Drawing for the job (mm, zero at the part's lowest x, y, z). A direction names the side the tool comes from. Give positions to 0.01 mm unless a question says otherwise; leave off trailing zeros. Loops run counter-clockwise (first coordinate to the right, second up) from the corner with the lowest first, then second, coordinate; pieces in that order, holes last. Notation, with made-up numbers: (67.25, 5.25) -> (71.25, 5.25) arc R22 ccw to (71.25, 18.25) -> close; hole circle Ø7 at (-2.75, 5.5). An arc over 180 degrees is marked (long way). Write item = value, one per line.
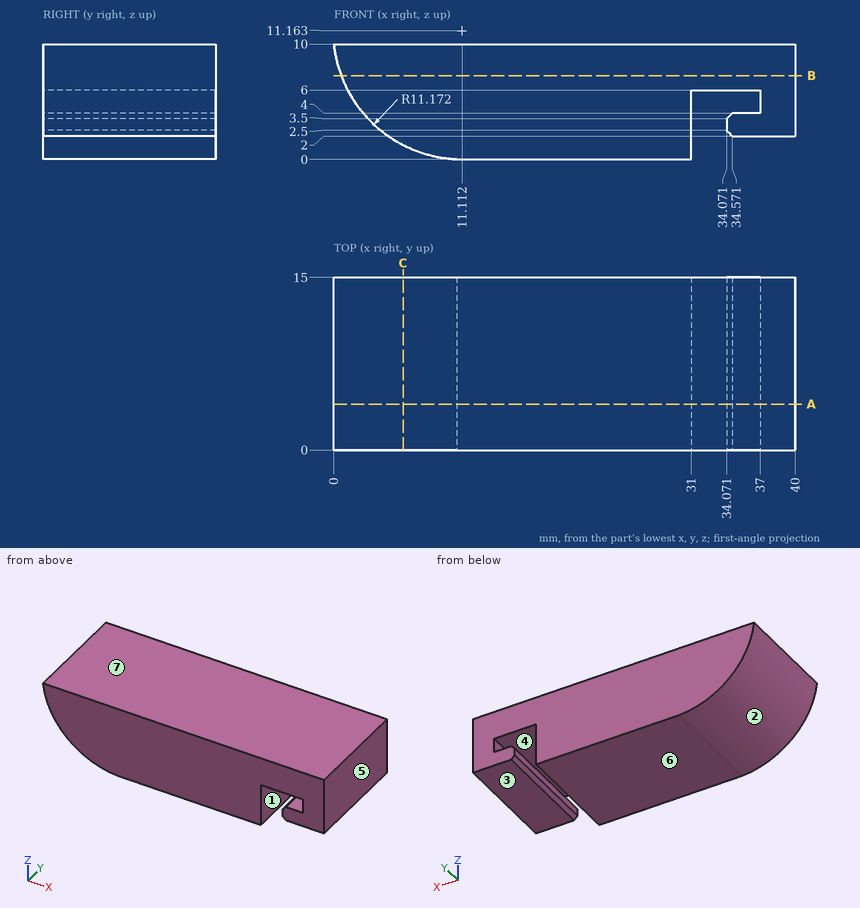
1) Pull direction Z, two halves, no side cores. Call the marked faces 4, 5, 6 and 7: pulls with the +Z half, pulls with the -Z half, needs draft (parallel to the pull), parting line crosses it, or undercut.
Resolved:
face_4 = undercut
face_5 = needs draft
face_6 = pulls with the -Z half
face_7 = pulls with the +Z half
2) Drop flat-ended pins along their axis: P1, Ø1.8, axis at x = 33, y = 10.5, coming from the -Z side; P2, Ø1, axis at y = 8.5, z = 4.5, coming from the -X side; P3, Ø0.5, axis at y = 5.5, z = 3, coming from the -X side (1 decimal). Give the stop position or say it passes through.
Resolved:
P1 = 6
P2 = 1.79
P3 = 3.2
3) Drill centre lines: line 1 along X through (y, z) = (1, 3.5); line 2 along Z through (x, y) = (37.5, 8.5); line 3 along X through (y, z) = (4.5, 4.75) (1 decimal). Where is each one in solid material? Low to high. Write a range as [from, to].
Resolved:
line_1 = [2.98, 31], [34.07, 40]
line_2 = [2, 10]
line_3 = [2, 31], [37, 40]
4) Slice it at B-B, the plane z = 7.25. List the corners of the cut face in (x, y), and give its area (3 significant figures).
Resolved:
outline = (0.65, 0) -> (40, 0) -> (40, 15) -> (0.65, 15) -> close
area = 590 mm²
5) Slice it at C-C, the plane x = 6. List the corners of the cut face in (y, z).
Resolved:
outline = (0, 1.23) -> (15, 1.23) -> (15, 10) -> (0, 10) -> close
6) Which spindle directions (+Z, -Z, +X, -X, +Y, -Y) get a long thin tool onto all of the face, cutting with end or side? Do the marked faces 1, 2 and 3. Say none if no direction does.
Resolved:
face_1 = -Z, +Y, -Y
face_2 = -Z, -X, +Y, -Y
face_3 = -Z, +X, +Y, -Y
7) Slice it at A-A, the plane y = 4. List the corners of the cut face in (x, z) (1 decimal).
Resolved:
outline = (0, 10) arc R11.2 ccw to (10.7, 0) -> (31, 0) -> (31, 6) -> (37, 6) -> (37, 4) -> (34.6, 4) -> (34.1, 3.5) -> (34.1, 2.5) -> (34.6, 2) -> (40, 2) -> (40, 10) -> close
